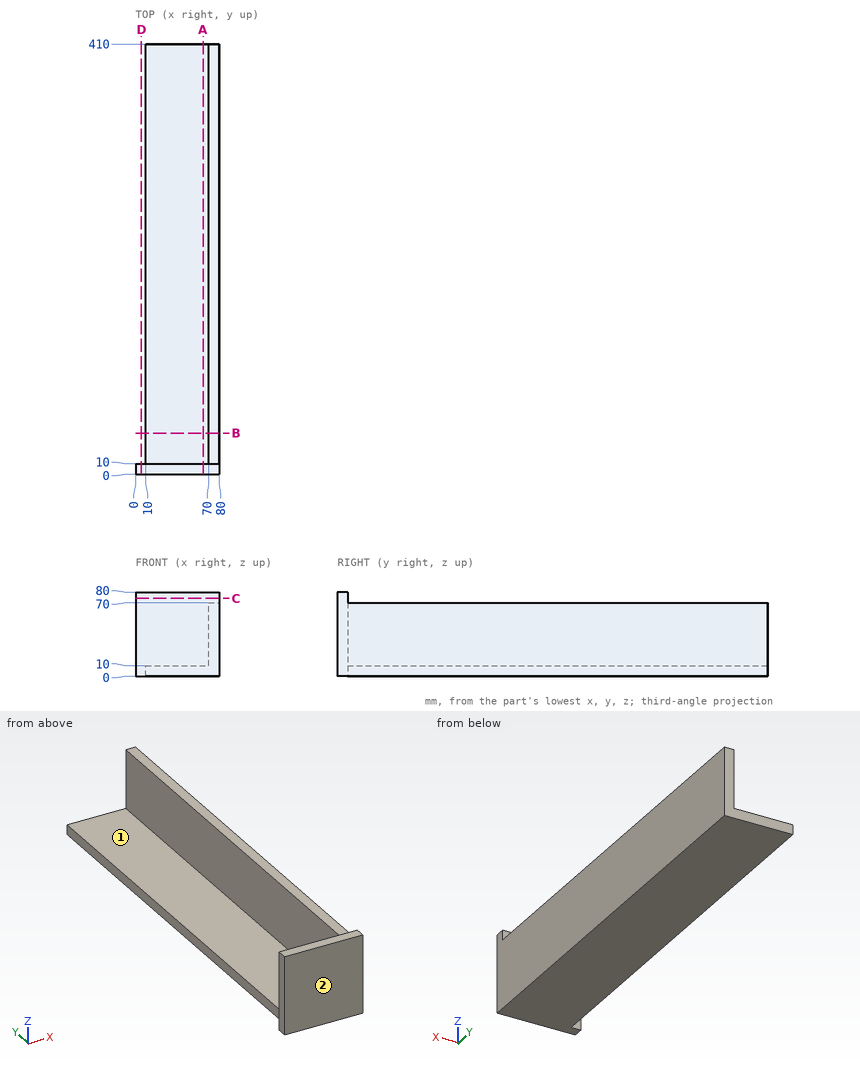
Part print with two shaded views. Sizes in mm from the minimum x, y, z corner. A direction names the side the tool comes from. Coordinates: 2 decimals unless noted, no trailing zeros. Write each loop counter-clockwise with the first axis right and the second up, starting at its lowest first coordinate (ties: lowest second). Pieces come first, ordered by that corner, then holes. Notation, with made-up numbers: (-35, 35) - (-9, 35) arc R17 cw to (-9, 52) - close; hole circle Ø9 at (-4.5, 44). An arc over 180 degrees is marked (long way). One line per item, written item: value. Start each with the question number.
1. Tool access for the marked faces 1 and 2: list every direction of +Z, -Z, +X, -X, +Y, -Y with a clear straight run to the whole face (end or side of a thin tool).
2. Slice it at D-D (x = 5.5). Write the cut outline in (y, z).
3. Probe line 1 (Y direction, x = 10, z = 63); line 2 (X direction, y = 138.5, z = 6.5). List the from-to ranges inside material, lowest first. Write a range as from..to.
4. Slice it at A-A (x = 64.5). Write the cut outline in (y, z).
5. Slice it at C-C (z = 74). Write the cut outline in (x, y).
6. Flat gauge pins, fed straight in: pin 1 (5 mm diameter, centred on x = 41.5, y = 77, fed in from +Z); pin 2 (5 mm diameter, centred on x = 22, z = 71, fed in from -Y); pin 3 (3 mm diameter, centred on y = 222, z = 3, fed in from -X); pin 4 (1 mm diameter, centred on x = 55, z = 23.5, fed in from +Y). Where does each tip first touch, or does it go through?
7. Slice it at B-B (y = 39). Write the cut outline in (x, z), plus the area to 3 significant figures.
Answers below:
1. face 1: +Z, -X, +Y
1. face 2: +Z, -Z, +X, -X, -Y
2. outline: (0, 0) - (10, 0) - (10, 80) - (0, 80) - close
3. line 1: y = 0..10
3. line 2: x = 10..80
4. outline: (0, 0) - (410, 0) - (410, 10) - (10, 10) - (10, 80) - (0, 80) - close
5. outline: (0, 0) - (80, 0) - (80, 10) - (0, 10) - close
6. pin 1: stops at z = 10
6. pin 2: stops at y = 0
6. pin 3: stops at x = 10
6. pin 4: stops at y = 10
7. outline: (10, 0) - (80, 0) - (80, 70) - (70, 70) - (70, 10) - (10, 10) - close
7. area: 1,300 mm^2
